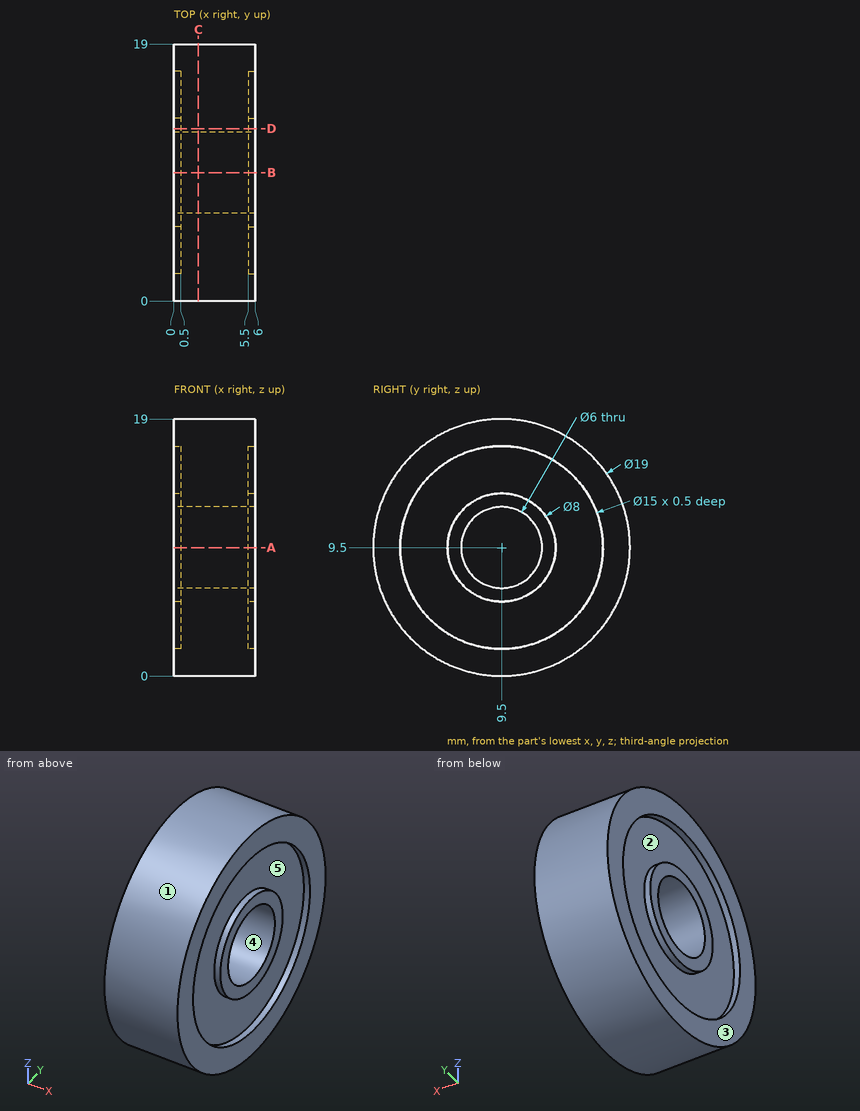
Geometry check sheet. Reference: drawing and pictorial views, mm from the part's lowest x, y, z. A direction names the side the tool comes from. Round coordinates to 2 decimals unless told otherwise and drop trailing zeros. Loops run counter-clockwise (first coordinate to the right, second up) from the corner with the lowest first, then second, coordinate; pieces in that order, holes last. Notation, with made-up numbers: (29, 76) - (40, 76) arc R11 ccw to (40, 93) - close; hole circle Ø7 at (4.25, 37.25). An arc over 180 degrees is marked (long way). Use a Markdown table: item, result.
Q1. Access from +Z, -Z, +X, -X, +Y, -Y to the whole of each face (thin tool, end or side, straight path). Record for the marked faces 4 and 5.
Solutions:
| item | result |
|---|---|
| face 4 | +X, -X |
| face 5 | +X |
Q2. Draft check along Z on the marked faces 1, 2 and 3. Enter one of: released by +Z, released by -Z, zero draft, split by the parting line, or undercut.
Solutions:
| item | result |
|---|---|
| face 1 | split by the parting line |
| face 2 | undercut |
| face 3 | zero draft |
Q3. Cross-section at A-A on z = 9.5. Record the cut outline in (x, y), plus the area to 3 significant figures.
Solutions:
| item | result |
|---|---|
| outline | (0, 0) - (6, 0) - (6, 2) - (5.5, 2) - (5.5, 5.5) - (6, 5.5) - (6, 6.5) - (0, 6.5) - (0, 5.5) - (0.5, 5.5) - (0.5, 2) - (0, 2) - close; (0, 12.5) - (6, 12.5) - (6, 13.5) - (5.5, 13.5) - (5.5, 17) - (6, 17) - (6, 19) - (0, 19) - (0, 17) - (0.5, 17) - (0.5, 13.5) - (0, 13.5) - close |
| area | 71.0 mm2 |
Q4. Go/stop test with flat-tipped pins: P1, Ø1, axis at x = 1.5, z = 5, coming from the -Y side; P2, Ø1.5, axis at y = 13.5, z = 3.5, coming from the +X side; P3, Ø3, axis at x = 5, z = 12, coming from the -Y side; P4, Ø1, axis at x = 2.5, y = 2.5, coming from the +Z side. Record where each tip stops, or that it passes through.
Solutions:
| item | result |
|---|---|
| P1 | stops at y = 0.88 |
| P2 | stops at x = 6 |
| P3 | stops at y = 0.05 |
| P4 | stops at z = 16.43 |
Q5. Cross-section at D-D on y = 12.75. Record the cut outline in (x, z), plus the area to 3 significant figures.
Solutions:
| item | result |
|---|---|
| outline | (0, 0.57) - (6, 0.57) - (6, 2.74) - (5.5, 2.74) - (5.5, 7.17) - (6, 7.17) - (6, 11.83) - (5.5, 11.83) - (5.5, 16.26) - (6, 16.26) - (6, 18.43) - (0, 18.43) - (0, 16.26) - (0.5, 16.26) - (0.5, 11.83) - (0, 11.83) - (0, 7.17) - (0.5, 7.17) - (0.5, 2.74) - (0, 2.74) - close |
| area | 98.3 mm2 |
Q6. Cross-section at C-C on x = 1.8. Record the cut outline in (y, z), plus the area to 3 significant figures.
Solutions:
| item | result |
|---|---|
| outline | circle Ø19 at (9.5, 9.5); hole circle Ø6 at (9.5, 9.5) |
| area | 255 mm2 |
Q7. Material ranges on line 1 (Z direction, x = 3.9, y = 9.5); line 2 (X direction, y = 6, z = 4.75); line 3 (Y direction, x = 3.25, z = 8.75), recorded low to high.
Solutions:
| item | result |
|---|---|
| line 1 | z = 0 to 6.5, 12.5 to 19 |
| line 2 | x = 0.5 to 5.5 |
| line 3 | y = 0.03 to 6.6, 12.4 to 18.97 |
